The model under review builds one solid part; all positions refer to its coordinate system, in mm. A direction names the side the tool comes from. Round coordinates to 2 decimals unless told otherwise and drop trailing zeros. Write each loop counter-clockwise with the first axis right and the second up, starting at its lowest first coordinate (ties: lowest second). Pieces come first, ordered by that corner, then holes. Notation, with made-up numbers: (59.25, 36.5) - (69.25, 36.5) arc R14 ccw to (69.25, 48.5) - close; hole circle Ø1 at (-30, 49.5). An arc over 180 degrees is marked (long way). Use one line per item in the form item = value.
from build123d import *

# Parameters (mm, degrees)
SCHIZZO1_W                     = 40
SCHIZZO1_H                     = 20
ESTRUSIONE_ESTRUSIONE1_DEPTH   = 20
TAGLIO_ESTRUSIONE1_DEPTH       = 20
FORO_PER_VITE_M1_1_D           = 1.3
FORO_PER_VITE_M1_1_CSINK_D     = 1.35
FORO_PER_VITE_M1_1_CSINK_ANGLE = 90
SPECCHIA2_COPY_1_D             = 1.3
SPECCHIA2_COPY_1_CSINK_D       = 1.35
SPECCHIA2_COPY_1_CSINK_ANGLE   = 90


with BuildPart() as part:
    # Schizzo1 → Estrusione-Estrusione1 (new body)
    with BuildSketch(Plane.XY):
        with Locations((20, 10)):
            Rectangle(SCHIZZO1_W, SCHIZZO1_H)
    extrude(amount=-ESTRUSIONE_ESTRUSIONE1_DEPTH)

    # Schizzo2 → Taglio-Estrusione1 (cut)
    with BuildSketch(Plane(origin=(0, 20, 0), x_dir=(1, 0, 0), z_dir=(0, 1, 0))):
        Polygon((4, 18), (4, 16), (2, 16), (2, 4), (4, 4), (4, 2), (36, 2), (36, 4), (38, 4), (38, 16), (36, 16), (36, 18), align=None)
    extrude(amount=-TAGLIO_ESTRUSIONE1_DEPTH, mode=Mode.SUBTRACT)

    # Sweep1: sweep along a path in Schizzo4
    with BuildLine(Plane(origin=(0, 20, 0), x_dir=(1, 0, 0), z_dir=(0, 1, 0))) as sweep1_path:
        Line((1, 19), (39, 19))
        Line((39, 19), (39, 1))
        Line((39, 1), (1, 1))
        Line((1, 1), (1, 19))
    # Schizzo3 → Sweep1 (sweep)
    with BuildSketch(Plane.XY.offset(-10)):
        with BuildLine():
            Line((0.75, 20), (1.25, 20))
            ThreePointArc((1.25, 20), (1, 20.25), (0.75, 20))
        make_face()
    sweep(path=sweep1_path.line, transition=Transition.RIGHT)

    # Taglia-Sweep1: sweep along a path in Schizzo5
    with BuildLine(Plane.XZ) as taglia_sweep1_path:
        Line((1, -19), (39, -19))
        Line((39, -19), (39, -1))
        Line((39, -1), (1, -1))
        Line((1, -1), (1, -19))
    # Schizzo6 → Taglia-Sweep1 (sweep, cut)
    with BuildSketch(Plane.XY.offset(-10)):
        with BuildLine():
            Line((0.75, 0), (1.25, 0))
            ThreePointArc((1.25, 0), (1, 0.25), (0.75, 0))
        make_face()
    sweep(path=taglia_sweep1_path.line, transition=Transition.RIGHT, mode=Mode.SUBTRACT)

    # Foro per Vite M1-1 (through all)
    with Locations(Plane(origin=(0, 0, 0), x_dir=(-1, 0, 0), z_dir=(0, -1, 0))):
        with Locations((-37.375, 17.375)):
            foro_per_vite_m1_1 = CounterSinkHole(FORO_PER_VITE_M1_1_D / 2, FORO_PER_VITE_M1_1_CSINK_D / 2, counter_sink_angle=FORO_PER_VITE_M1_1_CSINK_ANGLE)

    # Specchia1: Foro per Vite M1-1 across plane
    add(foro_per_vite_m1_1.mirror(Plane.XY.offset(-10)), mode=Mode.SUBTRACT)

    # Specchia2: Foro per Vite M1-1 across plane
    add(foro_per_vite_m1_1.mirror(Plane(origin=(20, 0, 0), x_dir=(0, 0, 1), z_dir=(1, 0, 0))), mode=Mode.SUBTRACT)

    # Specchia2 copy 1 (through all)
    with Locations(Plane(origin=(40, 0, -20), x_dir=(1, 0, 0), z_dir=(0, -1, 0))):
        with Locations((-37.375, 17.375)):
            CounterSinkHole(SPECCHIA2_COPY_1_D / 2, SPECCHIA2_COPY_1_CSINK_D / 2, counter_sink_angle=SPECCHIA2_COPY_1_CSINK_ANGLE)


solid = part.part
(1) To check wall thickness, follow L1, parallel to X at y = 4.25, z = -8.5; L2, parallel to X at y = 17.25, z = -3.75; L3, parallel to Z at x = 33, y = 17. State the ranges of each line that lie inside material, in increasing order.
Geometry results:
L1 = 0 to 2, 38 to 40
L2 = 0 to 4, 36 to 40
L3 = -20 to -18, -2 to 0
(2) The part is to be moulded in two halves that separate along Z. For faces 3 (the flat face through (15.7, 20, -1.5)), 4 (the flat face through (0, 10, -10)), 5 (the flat face through (2, 10, -10)), say which applies: +Z half, -Z half, draft (parallel to the pull), parting line (faces both ways), or undercut.
Geometry results:
face_3 = undercut
face_4 = draft
face_5 = undercut
(3) Insertion check: P1, Ø1.7, axis at x = 37.375, z = -17.375, coming from the +Y side. The pin has a flat end and moves straight along its axis. Give the tip position at first contact, or say it passes through.
Geometry results:
P1 = 20
(4) Add section A-A on x = 12. Write out the cut boundary in (y, z), then the cut area to 3 significant figures.
Geometry results:
outline = (0, -20) - (20, -20) - (20, -19.25) arc R0.25 ccw to (20, -18.75) - (20, -18) - (0, -18) - (0, -18.75) arc R0.25 cw to (0, -19.25) - close; (0, -2) - (20, -2) - (20, -1.25) arc R0.25 ccw to (20, -0.75) - (20, 0) - (0, 0) - (0, -0.75) arc R0.25 cw to (0, -1.25) - close
area = 80.0 mm2
(5) Add section B-B on z = -4.5. Write out the cut boundary in (x, y).
Geometry results:
outline = (0, 0) - (0.75, 0) arc R0.25 cw to (1.25, 0) - (2, 0) - (2, 20) - (1.25, 20) arc R0.25 ccw to (0.75, 20) - (0, 20) - close; (38, 0) - (38.75, 0) arc R0.25 cw to (39.25, 0) - (40, 0) - (40, 20) - (39.25, 20) arc R0.25 ccw to (38.75, 20) - (38, 20) - close
(6) Machinability: for faces 1 (the flat face through (15.7, 0, -18.4)), 2 (the flat face through (3, 10, -16)), which of the approach directions +Z, -Z, +X, -X, +Y, -Y give a long, thin tool a straight path to every point of the face, cutting with its end or side? Answer none if there is none.
Geometry results:
face_1 = +Z, -Z, +X, -X, -Y
face_2 = +Y, -Y
(7) Add section C-C on y = 12. Write out the cut boundary in (x, z) (3 decimals).
Geometry results:
outline = (0, -20) - (40, -20) - (40, 0) - (0, 0) - close; hole circle Ø1.3 at (2.625, -17.375); hole circle Ø1.3 at (2.625, -2.625); hole (2, -16) - (4, -16) - (4, -18) - (36, -18) - (36, -16) - (38, -16) - (38, -4) - (36, -4) - (36, -2) - (4, -2) - (4, -4) - (2, -4) - close; hole circle Ø1.3 at (37.375, -17.375); hole circle Ø1.3 at (37.375, -2.625)
